Model file for the job. Use its own axes, mm. A direction names the side the tool comes from. Coordinates: 2 decimals unless noted, no trailing zeros. Loops run counter-clockwise (first coordinate to the right, second up) from the corner with the lowest first, then second, coordinate; pieces in that order, holes last. Notation, with made-up numbers: (41.25, 1.5) -> (85.25, 1.5) arc R20 ccw to (85.25, 15.5) -> close; hole circle Ø4 at (-30.75, 27). An arc over 180 degrees is marked (long way). Use one line per item in the form item = value.
```python
from build123d import *
from OCP.BRepFilletAPI import BRepFilletAPI_MakeChamfer

# Parameters (mm, degrees)
SKETCH_1_W                  = 10
SKETCH_1_H                  = 15
SKETCH_6_R                  = 14
SKETCH_6_R_2                = 10
EXTRUDE_1_DEPTH             = 3
SKETCH_7_R                  = 19.5
EXTRUDE_2_DEPTH             = 10
EXTRUDE_START               = -10
EXTRUDE_3_DEPTH             = 10
EXTRUDE_4_DEPTH             = 10
HOLE_WIZARD_M43_D           = 3.3
HOLE_WIZARD_M43_DEPTH       = 10
HOLE_WIZARD_M43_CSINK_D     = 5
HOLE_WIZARD_M43_CSINK_ANGLE = 90
HOLE_WIZARD_M43_TIP         = 0.991420021
HOLE_WIZARD_M61_D           = 5
HOLE_WIZARD_M61_CSINK_D     = 7
HOLE_WIZARD_M61_CSINK_ANGLE = 90
HOLE_WIZARD_M62_D           = 5
HOLE_WIZARD_M62_CSINK_D     = 7
HOLE_WIZARD_M62_CSINK_ANGLE = 90
CHAMFER_1_SIZE              = 1
CHAMFER_2_SIZE              = 10
CHAMFER_2_SIZE2             = 10.916011313
FILLET_1_R                  = 10


with BuildPart() as part:
    # Эскиз1 → Повернуть1 (revolve)
    with BuildSketch(Plane.XY, mode=Mode.PRIVATE) as revolve_1_sk:
        with Locations((5, 21.5)):
            Rectangle(SKETCH_1_W, SKETCH_1_H)
    revolve(revolve_1_sk.sketch.rotate(Axis((-29.36512031, 0, 0), (1, 0, 0)), 90), axis=Axis((-29.36512031, 0, 0), (1, 0, 0)))

    # Эскиз6 → Бобышка-Вытянуть1 (add)
    with BuildSketch(Plane.ZY):
        Circle(SKETCH_6_R)
        Circle(SKETCH_6_R_2, mode=Mode.SUBTRACT)
    extrude(amount=-EXTRUDE_1_DEPTH)

    # Эскиз7 → Бобышка-Вытянуть2 (add)
    with BuildSketch(Plane.ZY):
        with BuildLine():
            Line((-42.192192379, -30), (42.192192379, -30))
            Line((42.192192379, -30), (25.406687144, 10.52379439))
            ThreePointArc((25.406687144, 10.52379439), (0, 27.5), (-25.406687144, 10.52379439))
            Line((-25.406687144, 10.52379439), (-42.192192379, -30))
        make_face()
        Circle(SKETCH_7_R, mode=Mode.SUBTRACT)
    extrude(amount=-EXTRUDE_2_DEPTH)

    # Эскиз10 → Бобышка-Вытянуть3 (add)
    with BuildSketch(Plane.ZY.offset(EXTRUDE_START)):
        with BuildLine():
            Line((-35.371237807, 14.27620235), (-28.740816158, 3.868525117))
            ThreePointArc((-28.740816158, 3.868525117), (-25.11473671, 14.5), (-17.720649105, 22.95601436))
            Line((-17.720649105, 22.95601436), (-30.049172808, 23.494289329))
            ThreePointArc((-30.049172808, 23.494289329), (-35.507041555, 20.5), (-35.371237807, 14.27620235))
        make_face()
        with BuildLine():
            Line((30.049172808, 23.494289329), (17.720649105, 22.95601436))
            ThreePointArc((17.720649105, 22.95601436), (25.11473671, 14.5), (28.740816158, 3.868525117))
            Line((28.740816158, 3.868525117), (35.371237807, 14.27620235))
            ThreePointArc((35.371237807, 14.27620235), (35.507041555, 20.5), (30.049172808, 23.494289329))
        make_face()
    extrude(amount=EXTRUDE_3_DEPTH)

    # Эскиз14 → Бобышка-Вытянуть4 (add)
    with BuildSketch(Plane(origin=(10, 0, 0), x_dir=(0, 0, -1), z_dir=(1, 0, 0))):
        with BuildLine():
            Line((-5.543277195, 37.296100594), (-9.666616005, 27.341480118))
            ThreePointArc((-9.666616005, 27.341480118), (0, 29), (9.666616005, 27.341480118))
            Line((9.666616005, 27.341480118), (5.543277195, 37.296100594))
            ThreePointArc((5.543277195, 37.296100594), (0, 41), (-5.543277195, 37.296100594))
        make_face()
    extrude(amount=-EXTRUDE_4_DEPTH)

    # Отверстие обработанное метчиком M43
    with Locations(Plane(origin=(0, -30, 0), x_dir=(-1, 0, 0), z_dir=(0, -1, 0))):
        with Locations((-5, 0), (-5, 25), (-5, -25)):
            CounterSinkHole(HOLE_WIZARD_M43_D / 2, HOLE_WIZARD_M43_CSINK_D / 2, depth=HOLE_WIZARD_M43_DEPTH, counter_sink_angle=HOLE_WIZARD_M43_CSINK_ANGLE)
            with Locations((0, 0, -(HOLE_WIZARD_M43_DEPTH + HOLE_WIZARD_M43_TIP / 2))):  # 118° drill point
                Cone(0, HOLE_WIZARD_M43_D / 2, HOLE_WIZARD_M43_TIP, mode=Mode.SUBTRACT)

    # Отверстие обработанное метчиком M61 (through all)
    with Locations(Plane(origin=(0, 0, 0), x_dir=(0, 0, -1), z_dir=(-1, 0, 0))):
        with Locations((30.310889132, -17.5), (-30.310889132, -17.5), (-30.310889132, 17.5), (30.310889132, 17.5)):
            CounterSinkHole(HOLE_WIZARD_M61_D / 2, HOLE_WIZARD_M61_CSINK_D / 2, counter_sink_angle=HOLE_WIZARD_M61_CSINK_ANGLE)

    # Отверстие обработанное метчиком M62 (through all)
    with Locations(Plane(origin=(10, 0, 0), x_dir=(0, 0, -1), z_dir=(1, 0, 0))):
        with Locations((0, 35)):
            CounterSinkHole(HOLE_WIZARD_M62_D / 2, HOLE_WIZARD_M62_CSINK_D / 2, counter_sink_angle=HOLE_WIZARD_M62_CSINK_ANGLE)

    # Фаска1
    chamfer_1_edges = [part.edges().sort_by_distance(p)[0] for p in [
        (10, 0, -14),
    ]]
    chamfer(chamfer_1_edges, length=CHAMFER_1_SIZE)

    # Фаска2: one chamfer whose edges measure the first distance from different faces: ONE call of the kernel's chamfer builder (chamfer() names one face for all edges)
    chamfer_2_edges_1 = [part.edges().sort_by_distance(p)[0] for p in [
        (5, -30, -42.192192379),
    ]]
    chamfer_2_side_1 = [part.faces().sort_by_distance(p)[0] for p in [
        (5, -30, -41.342443923),
    ]]
    chamfer_2_edges_2 = [part.edges().sort_by_distance(p)[0] for p in [
        (5, -30, 42.192192379),
    ]]
    chamfer_2_side_2 = [part.faces().sort_by_distance(p)[0] for p in [
        (5, -13.990709354, 35.56092707),
    ]]
    chamfer_2 = BRepFilletAPI_MakeChamfer(part.part.solid().wrapped)
    for e in chamfer_2_edges_1:
        chamfer_2.Add(CHAMFER_2_SIZE, CHAMFER_2_SIZE2, e.wrapped, chamfer_2_side_1[0].wrapped)  # the first distance lies on this face
    for e in chamfer_2_edges_2:
        chamfer_2.Add(CHAMFER_2_SIZE, CHAMFER_2_SIZE2, e.wrapped, chamfer_2_side_2[0].wrapped)  # the first distance lies on this face
    add(Compound.cast(chamfer_2.Shape()), mode=Mode.REPLACE)

    # Скругление1
    fillet_1_edges = [part.edges().sort_by_distance(p)[0] for p in [
        (5, -20.761204675, 38.365358056),
        (5, -19.914920571, -38.014815702),
    ]]
    fillet(fillet_1_edges, radius=FILLET_1_R)


solid = part.part
```
Q1. Wall check: line 1 along Z through (x, y) = (5.5, 17.5); line 2 along Y through (x, z) = (0.7, 0); line 3 along X through (y, z) = (-24.5, 25). Give the ranges that are in metal, low to high.
Result:
line_1 = -36.31 to -32.81, -27.81 to 27.81, 32.81 to 36.31
line_2 = -30 to -10, 10 to 32.5, 37.5 to 41
line_3 = 0 to 3.35, 6.65 to 10
Q2. Band-saw the part on C-C, the plane z = -16.5. Write the cut outline in (x, y), and give its area (3 significant figures).
Result:
outline = (0, -30) -> (10, -30) -> (10, 23.85) -> (0, 23.85) -> close
area = 538 mm2
Q3. Pin check, flat tips, straight feed: pin 1 Ø1 at (x, z) = (7.5, 3.5) entering from +Y; pin 2 Ø2.5 at (x, z) = (5, 0) entering from -Y; pin 3 Ø1.5 at (x, y) = (5.5, -13) entering from +Z. Stop position of each tip, or through.
Result:
pin_1 = 40.2
pin_2 = -19.76
pin_3 = 35.46
Q4. Band-saw the part on B-B, the plane y = 35. Write the cut outline in (x, z).
Result:
outline = (0, -6.49) -> (10, -6.49) -> (10, -3.5) -> (9, -2.5) -> (0, -2.5) -> close; (0, 2.5) -> (9, 2.5) -> (10, 3.5) -> (10, 6.49) -> (0, 6.49) -> close
Q5. Band-saw the part on A-A, the plane y = 17.5. Write the cut outline in (x, z), and give its area (3 significant figures).
Result:
outline = (0, -36.31) -> (10, -36.31) -> (10, -32.81) -> (1, -32.81) -> (0, -33.81) -> close; (0, -26.81) -> (1, -27.81) -> (10, -27.81) -> (10, 27.81) -> (1, 27.81) -> (0, 26.81) -> close; (0, 33.81) -> (1, 32.81) -> (10, 32.81) -> (10, 36.31) -> (0, 36.31) -> close
area = 624 mm2
Q6. Mould opens along Y. For faces 4 (the face through (2, -30, -1)), 5 (the face through (3.35, -24.51, -0.07)), 6 (the face through (5.563, -17.61, 27.813)), 7 (the face through (5.07, 25.44, -13.92)) say: released by +Y, released by -Y, zero draft, split by the parting line, or undercut.
Result:
face_4 = released by -Y
face_5 = zero draft
face_6 = undercut
face_7 = released by +Y
Q7. Which spindle directions (+Z, -Z, +X, -X, +Y, -Y) get a long thin tool onto all of the face, cutting with end or side? Do faces 1 (the face through (4.93, -6.55, -32.48)), 2 (the face through (6, 12.4, 6.5)), 3 (the face through (4.785, -24.511, -26.636)). Say none if no direction does.
Result:
face_1 = -Z, +X, -X
face_2 = +X
face_3 = -Y
